from build123d import *

# Parameters (mm, degrees)
ESBO_O1_R                = 1.6
RESSALTO_EXTRUS_O1_DEPTH = 4
RESSALTO_EXTRUS_O2_DEPTH = 4


with BuildPart() as part:
    # Esbo_o1 → Ressalto-extrus_o1 (new body)
    with BuildSketch(Plane.XY):
        with BuildLine():
            Line((-5.428931338, -10.411256864), (-4.040153116, -8.653603149))
            ThreePointArc((-4.040153116, -8.653603149), (-3.651813796, -8.395770502), (-3.186165661, -8.417146095))
            ThreePointArc((-3.186165661, -8.417146095), (-2.535977815, -8.635323765), (-1.871064211, -8.803358377))
            ThreePointArc((-1.871064211, -8.803358377), (-1.465141223, -9.040151498), (-1.27980553, -9.472002324))
            Line((-1.27980553, -9.472002324), (-1.087391415, -11.684866251))
            ThreePointArc((-1.087391415, -11.684866251), (-0.855086446, -12.165243662), (-0.362160028, -12.369575749))
            ThreePointArc((-0.362160028, -12.369575749), (-0.013315066, -12.374869163), (0.335540479, -12.370326458))
            ThreePointArc((0.335540479, -12.370326458), (0.826548297, -12.16926195), (1.061642754, -11.693608494))
            Line((1.061642754, -11.693608494), (1.279697998, -9.464145904))
            ThreePointArc((1.279697998, -9.464145904), (1.466994971, -9.037291191), (1.870279627, -8.803525096))
            ThreePointArc((1.870279627, -8.803525096), (2.535208203, -8.635549743), (3.185415492, -8.41743002))
            ThreePointArc((3.185415492, -8.41743002), (3.654919666, -8.397174533), (4.044310156, -8.660270526))
            Line((4.044310156, -8.660270526), (5.402543773, -10.417823198))
            ThreePointArc((5.402543773, -10.417823198), (5.857682784, -10.696348844), (6.382829142, -10.601747792))
            ThreePointArc((6.382829142, -10.601747792), (6.679158034, -10.41760107), (6.970178022, -10.225173956))
            ThreePointArc((6.970178022, -10.225173956), (7.274536404, -9.790568861), (7.215152773, -9.263322051))
            Line((7.215152773, -9.263322051), (6.19325404, -7.269889205))
            ThreePointArc((6.19325404, -7.269889205), (6.120043199, -6.809535782), (6.332924348, -6.394847082))
            ThreePointArc((6.332924348, -6.394847082), (6.80148353, -5.894049694), (7.230548283, -5.359027107))
            ThreePointArc((7.230548283, -5.359027107), (7.614569385, -5.088153986), (8.084385943, -5.098964027))
            Line((8.084385943, -5.098964027), (10.177209485, -5.843194888))
            ThreePointArc((10.177209485, -5.843194888), (10.710679119, -5.831438844), (11.101315158, -5.46793982))
            ThreePointArc((11.101315158, -5.46793982), (11.251045651, -5.152818244), (11.391833292, -4.833600971))
            ThreePointArc((11.391833292, -4.833600971), (11.412910602, -4.303439334), (11.077902766, -3.891996308))
            Line((11.077902766, -3.891996308), (9.140495683, -2.76749405))
            ThreePointArc((9.140495683, -2.76749405), (8.830020954, -2.419800875), (8.784910335, -1.955850303))
            ThreePointArc((8.784910335, -1.955850303), (8.908335893, -1.281230512), (8.980033083, -0.599170952))
            ThreePointArc((8.980033083, -0.599170952), (9.156647127, -0.163680499), (9.557726315, 0.081227523))
            Line((9.557726315, 0.081227523), (11.720683094, 0.586606513))
            ThreePointArc((11.720683094, 0.586606513), (12.163110512, 0.884911785), (12.295212049, 1.401900411))
            ThreePointArc((12.295212049, 1.401900411), (12.25080577, 1.747947966), (12.196661982, 2.09260617))
            ThreePointArc((12.196661982, 2.09260617), (11.927766323, 2.550001774), (11.423496904, 2.715010763))
            Line((11.423496904, 2.715010763), (9.185694531, 2.613560912))
            ThreePointArc((9.185694531, 2.613560912), (8.736529446, 2.738203711), (8.447749362, 3.104115127))
            ThreePointArc((8.447749362, 3.104115127), (8.186854553, 3.738370305), (7.878420829, 4.350917747))
            ThreePointArc((7.878420829, 4.350917747), (7.791554103, 4.812760389), (7.996556113, 5.235629909))
            Line((7.996556113, 5.235629909), (9.542922635, 6.83016449))
            ThreePointArc((9.542922635, 6.83016449), (9.753840257, 7.320309176), (9.585465989, 7.826647167))
            ThreePointArc((9.585465989, 7.826647167), (9.361021617, 8.093753047), (9.129136671, 8.354425638))
            ThreePointArc((9.129136671, 8.354425638), (8.655640515, 8.593835336), (8.142211489, 8.4600211))
            Line((8.142211489, 8.4600211), (6.314500268, 7.16482875))
            ThreePointArc((6.314500268, 7.16482875), (5.869251568, 7.026847967), (5.428487655, 7.178545938))
            ThreePointArc((5.428487655, 7.178545938), (4.866104738, 7.571064963), (4.275465628, 7.919620803))
            ThreePointArc((4.275465628, 7.919620803), (3.952697704, 8.26118386), (3.896535847, 8.727756791))
            Line((3.896535847, 8.727756791), (4.335351667, 10.905193502))
            ThreePointArc((4.335351667, 10.905193502), (4.247794638, 11.431560125), (3.832402205, 11.766488747))
            ThreePointArc((3.832402205, 11.766488747), (3.499179242, 11.869848724), (3.16317497, 11.963773995))
            ThreePointArc((3.16317497, 11.963773995), (2.635410001, 11.909186901), (2.275831457, 11.519034514))
            Line((2.275831457, 11.519034514), (1.438496786, 9.441314085))
            ThreePointArc((1.438496786, 9.441314085), (1.138527788, 9.084517642), (0.685719474, 8.973839134))
            ThreePointArc((0.685719474, 8.973839134), (0.000401051, 8.999999991), (-0.684919701, 8.973900211))
            ThreePointArc((-0.684919701, 8.973900211), (-1.141112287, 9.086739826), (-1.440607019, 9.44888256))
            Line((-1.440607019, 9.44888256), (-2.248662823, 11.517900629))
            ThreePointArc((-2.248662823, 11.517900629), (-2.606895765, 11.913371507), (-3.137422201, 11.970553289))
            ThreePointArc((-3.137422201, 11.970553289), (-3.473627818, 11.877351299), (-3.807072434, 11.774708641))
            ThreePointArc((-3.807072434, 11.774708641), (-4.221544568, 11.44345577), (-4.313108983, 10.920835859))
            Line((-4.313108983, 10.920835859), (-3.894219261, 8.720248907))
            ThreePointArc((-3.894219261, 8.720248907), (-3.953670521, 8.257917155), (-4.274759795, 7.920001811))
            ThreePointArc((-4.274759795, 7.920001811), (-4.865429967, 7.571498612), (-5.427847864, 7.179029709))
            ThreePointArc((-5.427847864, 7.179029709), (-5.87262719, 7.0273201), (-6.320367336, 7.170054878))
            Line((-6.320367336, 7.170054878), (-8.118742756, 8.473755688))
            ThreePointArc((-8.118742756, 8.473755688), (-8.633915182, 8.612771611), (-9.111137226, 8.374051741))
            ThreePointArc((-9.111137226, 8.374051741), (-9.343582589, 8.113878758), (-9.56860124, 7.847256489))
            ThreePointArc((-9.56860124, 7.847256489), (-9.738188564, 7.344508289), (-9.532667795, 6.855348982))
            Line((-9.532667795, 6.855348982), (-7.990548209, 5.230566315))
            ThreePointArc((-7.990548209, 5.230566315), (-7.790606374, 4.809486318), (-7.878033033, 4.351619874))
            ThreePointArc((-7.878033033, 4.351619874), (-8.186521347, 3.739099922), (-8.447472682, 3.104867999))
            ThreePointArc((-8.447472682, 3.104867999), (-8.739624454, 2.736775896), (-9.19345568, 2.614785434))
            Line((-9.19345568, 2.614785434), (-11.411179228, 2.739253189))
            ThreePointArc((-11.411179228, 2.739253189), (-11.919727533, 2.577677583), (-12.192130558, 2.118847933))
            ThreePointArc((-12.192130558, 2.118847933), (-12.247015907, 1.774307042), (-12.292166761, 1.428355848))
            ThreePointArc((-12.292166761, 1.428355848), (-12.163026498, 0.913731319), (-11.725671937, 0.61333724))
            Line((-11.725671937, 0.61333724), (-9.549934558, 0.080215876))
            ThreePointArc((-9.549934558, 0.080215876), (-9.15407975, -0.165922443), (-8.980086447, -0.598370627))
            ThreePointArc((-8.980086447, -0.598370627), (-8.908450044, -1.280436574), (-8.78508461, -1.955067363))
            ThreePointArc((-8.78508461, -1.955067363), (-8.831852706, -2.422675318), (-9.147686805, -2.77065991))
            Line((-9.147686805, -2.77065991), (-11.080646922, -3.864942843))
            ThreePointArc((-11.080646922, -3.864942843), (-11.421110614, -4.275810864), (-11.402208583, -4.809075122))
            ThreePointArc((-11.402208583, -4.809075122), (-11.262108208, -5.128594624), (-11.113056187, -5.444037682))
            ThreePointArc((-11.113056187, -5.444037682), (-10.726189458, -5.807148888), (-10.195858089, -5.823404741))
            Line((-10.195858089, -5.823404741), (-8.077284162, -5.095602537))
            ThreePointArc((-8.077284162, -5.095602537), (-7.611197484, -5.088652), (-7.231025864, -5.358382681))
            ThreePointArc((-7.231025864, -5.358382681), (-6.802008795, -5.893443506), (-6.333494247, -6.394282651))
            ThreePointArc((-6.333494247, -6.394282651), (-6.120030126, -6.812944237), (-6.197592003, -7.27644031))
            Line((-6.197592003, -7.27644031), (-7.232087511, -9.242046831))
            ThreePointArc((-7.232087511, -9.242046831), (-7.296371772, -9.771759573), (-6.992165948, -10.210150805))
            ThreePointArc((-6.992165948, -10.210150805), (-6.701560727, -10.403203734), (-6.405628795, -10.587987714))
            ThreePointArc((-6.405628795, -10.587987714), (-5.883863054, -10.684300355), (-5.428931338, -10.411256864))
        make_face()
        Circle(ESBO_O1_R, mode=Mode.SUBTRACT)
    extrude(amount=RESSALTO_EXTRUS_O1_DEPTH)

    # Esbo_o6 → Ressalto-extrus_o2 (add)
    with BuildSketch(Plane.XY.offset(4)):
        with BuildLine():
            Line((0, 12.37), (0, 9))
            ThreePointArc((0, 9), (6.887269468, 5.79357569), (8.867092658, -1.540995716))
            Line((8.867092658, -1.540995716), (12.192130558, -2.118847933))
            ThreePointArc((12.192130558, -2.118847933), (19.845997755, 27.157089417), (0, 50))
            ThreePointArc((0, 50), (7.793428176, 31.185), (0, 12.37))
        make_face()
    extrude(amount=-RESSALTO_EXTRUS_O2_DEPTH)


solid = part.part
Design review of the part built by this model. Coordinates are the model's own, in mm. A direction names the side the tool comes from. Coordinates: 2 decimals unless noted, no trailing zeros. Write each loop counter-clockwise with the first axis right and the second up, starting at its lowest first coordinate (ties: lowest second). Pieces come first, ordered by that corner, then holes. Notation, with made-up numbers: (-36, 30) - (4, 30) arc R27 ccw to (4, 59) - close; hole circle Ø6 at (-32.5, 69.25). An arc over 180 degrees is marked (long way). One line per item, written item: value.
1) Mouldability with a two-part tool opening along X and no side actions: class faces 1 (the face through (-8.77, 6.05, 1.97)), 2 (the face through (19.943, 26.727, 2.028)), 3 (the face through (-1.27, -0.97, 1.97)) as +X half, -X half, draft (parallel to the pull), parting line (faces both ways), or undercut.
Answer sheet:
face 1: -X half
face 2: +X half
face 3: undercut
2) Insertion check: pin 1 (1.5 mm diameter, centred on x = 2.5, z = 1.5, fed in from +Y); pin 2 (10 mm diameter, centred on x = 1.5, y = 19, fed in from +Z). Each pin has a flat end and moves straight along its axis. Give the tip position at first contact, or say it passes through.
Answer sheet:
pin 1: stops at y = 49.26
pin 2: stops at z = 4
3) Add section A-A (y = 15). State the section outline as (x, z) points (3 decimals).
Answer sheet:
outline: (2.305, 0) - (20.345, 0) - (20.345, 4) - (2.305, 4) - close
4) To check wall thickness, follow probe 1 along Y at (x, z) = (2.5, 0.95); probe 2 along Y at (x, z) = (5, 2.1); probe 3 along X at (y, z) = (8, 1.1). State the ranges of each line that lie inside material, in increasing order.
Answer sheet:
probe 1: y = -8.65 to 15.26, 47.11 to 48.91
probe 2: y = -9.9 to 19.32, 43.05 to 47.55
probe 3: x = -9.44 to -7.47, -4.16 to 18.49
5) Add section B-B (y = 35.5). State the section outline as (x, z) points.
Answer sheet:
outline: (7.44, 0) - (16.63, 0) - (16.63, 4) - (7.44, 4) - close
6) For faces 4 (the face through (-10.287, 2.676, 1.972)), 5 (the face through (1.17, -10.59, 1.97)), 6 (the face through (0, 11, 2)), list the 3-axis set-ups (+Z, -Z, +X, -X, +Y, -Y) from which the entire face can be reached by the end or side of a thin tool; tool diameter is ignored.
Answer sheet:
face 4: +Z, -Z
face 5: +Z, -Z, -Y
face 6: +Z, -Z, +Y
